Could you check a few things on this model? Use its own coordinates, in mm. Face numbers are marked on the shaded views. A direction names the side the tool comes from. Round coordinates to 2 decimals unless told otherwise and drop trailing zeros. One line per item, written item: value.
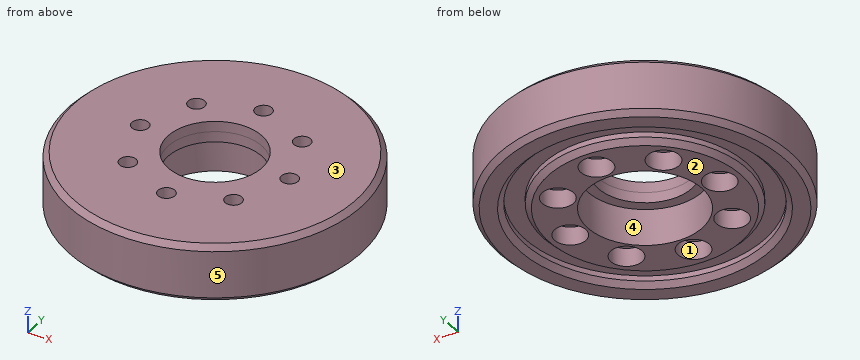
Autodesk Inventor part; units mm, degrees
ref_plane "YZ Plane" through (0, 0, 0) normal (1, 0, 0) x (0, 1, 0)
ref_plane "XZ Plane" through (0, 0, 0) normal (0, 1, 0) x (-1, 0, 0)
ref_plane "XY Plane" through (0, 0, 0) normal (0, 0, 1) x (1, 0, 0)
sketch "草图1" plane through (0, 0, 0) normal (0, 0, 1) x (1, 0, 0)
  circle A0 centre (0, 0) radius 28
  circle A1 centre (0, 0) radius 11
  dimension "d0" = 56
  dimension "d1" = 22
extrude "拉伸1" add sketch "草图1" along normal blind 9
sketch "草图2" plane through (0, 0, 9) normal (0, 0, 1) x (1, 0, 0)
  circle A0 centre (0, 0) radius 28
  circle A1 centre (0, 0) radius 9
  dimension "d4" = 18
extrude "拉伸2" add sketch "草图2" along normal blind 2
sketch "草图3" plane through (0, 0, 11) normal (0, 0, 1) x (1, 0, 0)
  circle A0 centre (0, 0) radius 14.5 construction
  line L0 (-36.9419, 0) -> (43.6936, 0) construction
  circle A1 centre (14.5, 0) radius 1.6
  circle A2 centre (10.253, 10.253) radius 1.6
  circle A3 centre (0, 14.5) radius 1.6
  circle A4 centre (-10.253, 10.253) radius 1.6
  circle A5 centre (-14.5, 0) radius 1.6
  circle A6 centre (-10.253, -10.253) radius 1.6
  circle A7 centre (0, -14.5) radius 1.6
  circle A8 centre (10.253, -10.253) radius 1.6
  dimension "d7" = 29
  dimension "d8" = 3.2
  dimension "d11" = 360
extrude "拉伸3" cut sketch "草图3" against normal through all
chamfer "倒角1" distance 1 angle 45 2 edges at (-28, 0, 0) (-28, 0, 11)
sketch "草图4" plane through (0, 0, 0) normal (0, 0, -1) x (-1, 0, 0)
  circle A0 centre (0, 0) radius 19.5
  circle A1 centre (0, 0) radius 23
  dimension "d18" = 39
  dimension "d19" = 46
extrude "拉伸4" cut sketch "草图4" against normal blind 2
chamfer "倒角2" distance 1 angle 45 2 edges at (23, 0, 0) (19.5, 0, 0)
sketch "草图5" plane through (0, 0, 0) normal (0, 0, -1) x (-1, 0, 0)
  circle A0 centre (0, 14.5) radius 1.6
  circle A1 centre (0, 14.5) radius 3
  circle A2 centre (-10.253, 10.253) radius 3
  circle A3 centre (-14.5, 0) radius 3
  circle A4 centre (-10.253, -10.253) radius 3
  circle A5 centre (0, -14.5) radius 3
  circle A6 centre (10.253, -10.253) radius 3
  circle A7 centre (14.5, 0) radius 3
  circle A8 centre (10.253, 10.253) radius 3
  point P0 (0, 0)
  dimension "d25" = 6
  dimension "d28" = 360
extrude "拉伸5" cut sketch "草图5" against normal blind 3.5
sketch "草图6" plane through (0, 0, 9) normal (0, 0, -1) x (-1, 0, 0)
  circle A0 centre (0, 0) radius 9
  circle A1 centre (0, 0) radius 11
extrude "拉伸6" add sketch "草图6" along normal blind 2
properties part number "内轮"
Item 1: If we mould it in two halves opening along X, with no side actions, what happens to the marked faces 3, 4 and 5? For each: released by +X, released by -X, zero draft, split by the parting line, or undercut.
Output:
face 3: zero draft
face 4: undercut
face 5: split by the parting line
Item 2: For the marked faces 1 and 2, which set-ups out of +Z, -Z, +X, -X, +Y, -Y let a thin tool reach every point of the face, with its end or its side?
Output:
face 1: -Z
face 2: -Z, +X, -X, +Y, -Y
Item 3: I need wall thicknesses on line 1 (Y direction, x = 0, z = 9.85); line 2 (Y direction, x = 0, z = 6.5); line 3 (Y direction, x = -7.5, z = 0.75). Which ranges of each line are inside material? Lowest first, please. Write a range as from..to.
Output:
line 1: y = -28..-16.1, -12.9..-9, 9..12.9, 16.1..28
line 2: y = -28..-16.1, -12.9..-11, 11..12.9, 16.1..28
line 3: y = -26.72..-22.01, -17.73..-11.45, -9.06..-8.05, 8.05..9.06, 11.45..17.73, 22.01..26.72
Item 4: If we section it at A-A on z = 5.5: Count the separate pieces of the cut face and the enclosed holes in it, plus the area to 3 significant figures.
Output:
separate pieces: 1
enclosed holes: 9
area: 2,020 mm²
Item 5: Will these pins go through, and if not, where does the flat tip stop? pin 1 Ø5 at (x, y) = (-10.253, -10.253) entering from +Z; pin 2 Ø6 at (y, z) = (8, 1.5) entering from -X; pin 3 Ø5 at (x, z) = (10, 4) entering from -Y; pin 4 Ø3 at (x, y) = (3, 20) entering from -Z.
Output:
pin 1: stops at z = 11
pin 2: stops at x = -27.55
pin 3: stops at y = -26.98
pin 4: stops at z = 0.22
